Verification items for the finished model (mm, model axes). Face numbers are marked on the shaded views. Coordinates: 2 decimals unless noted, no trailing zeros. Order: outer loops, then holes, each group sorted by start corner. A loop starts at its lowest first (then second) coordinate and runs counter-clockwise, first axis right, second up. Notation, with made-up numbers: (-3.75, 73.25) - (47.25, 73.25) arc R6 ccw to (47.25, 82.25) - close; hole circle Ø2 at (74, 80.5). An arc over 180 degrees is marked (long way). One line per question, with ' | ' between items. Start each with the question number.
from build123d import *

# Parameters (mm, degrees)
SKETCH1_W           = 160
SKETCH1_H           = 22
BOSS_EXTRUDE1_DEPTH = 1.25
SKETCH2_W           = 160
SKETCH2_H           = 2.5
BOSS_EXTRUDE2_DEPTH = 4.5
SKETCH4_R           = 1.6
CUT_EXTRUDE1_DEPTH  = 3.5


with BuildPart() as part:
    # Sketch1 → Boss-Extrude1 (new body, symmetric)
    with BuildSketch(Plane(origin=(0, 0, 0), x_dir=(1, 0, 0), z_dir=(0, 1, 0))):
        with Locations((-1.081081081, -6.855855856)):
            Rectangle(SKETCH1_W, SKETCH1_H)
    extrude(amount=BOSS_EXTRUDE1_DEPTH, both=True)

    # Sketch2 → Boss-Extrude2 (add)
    with BuildSketch(Plane(origin=(0, 1.25, 0), x_dir=(1, 0, 0), z_dir=(0, 1, 0))):
        with Locations((-1.081081081, 2.894144144)):
            Rectangle(SKETCH2_W, SKETCH2_H)
        with Locations((-1.081081081, -16.605855856)):
            Rectangle(SKETCH2_W, SKETCH2_H)
    extrude(amount=BOSS_EXTRUDE2_DEPTH)

    # Sketch4 → Cut-Extrude1 (cut, through all)
    with BuildSketch(Plane(origin=(0, 1.25, 0), x_dir=(1, 0, 0), z_dir=(0, 1, 0))):
        with Locations((73.918918919, -3.355855856)):
            Circle(SKETCH4_R)
        with Locations((73.918918919, -10.355855856)):
            Circle(SKETCH4_R)
        with Locations((-76.081081081, -10.355855856)):
            Circle(SKETCH4_R)
        with Locations((-76.081081081, -3.355855856)):
            Circle(SKETCH4_R)
    extrude(amount=-CUT_EXTRUDE1_DEPTH, mode=Mode.SUBTRACT)


solid = part.part
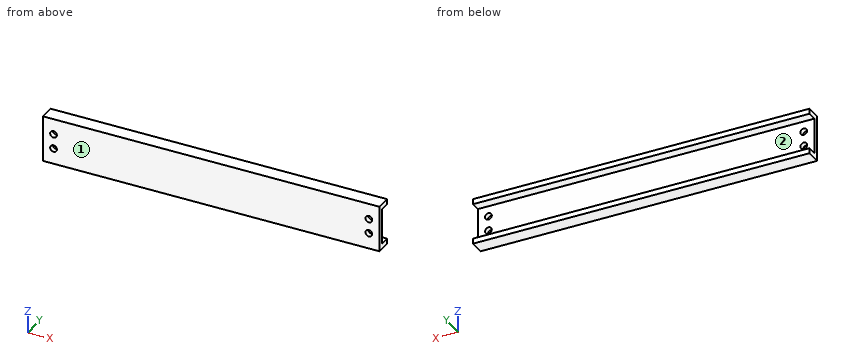
Item 1: Section check B-B (x = 60.5). Record the cut outline in (y, z), then the cut area to 3 significant figures.
Item 2: Section check C-C (z = 0). Record the cut outline in (x, y), then the cut area to 3 significant figures.
Item 3: Gauge pin test, flat end, axial feed: pin 1 (5 mm diameter, centred on x = 27, z = 3, fed in from +Y). Record the tip position at first contact, or that the pin passes through.
Item 4: Mould release check, pull along Z, two halves, no side actions. Record for the marked faces 1 and 2: +Z half, -Z half, draft (parallel to the pull), parting line (faces both ways), or undercut.
Item 5: Section check A-A (y = 4.25). Record the cut outline in (x, z), then the cut area to 3 significant figures.
Item 6: Thickness scan on probe 1 along X at (y, z) = (0.75, 3.25); probe 2 along Z at (x, y) = (-59, 1.5); probe 3 along X at (y, z) = (-0.5, 11.5). Record the ranges inside material, lowest first. Write a range as from..to.
Completed:
1) outline: (-1.25, -4.14) - (5.75, -4.14) - (5.75, -1.64) - (1.25, -1.64) - (1.25, 15.36) - (5.75, 15.36) - (5.75, 17.86) - (-1.25, 17.86) - close | area: 77.5 mm^2
2) outline: (-81.08, -1.25) - (78.92, -1.25) - (78.92, 1.25) - (-81.08, 1.25) - close | area: 400 mm^2
3) pin 1: stops at y = 1.25
4) face 1: draft | face 2: undercut
5) outline: (-81.08, -4.14) - (78.92, -4.14) - (78.92, -1.64) - (-81.08, -1.64) - close; (-81.08, 15.36) - (78.92, 15.36) - (78.92, 17.86) - (-81.08, 17.86) - close | area: 800 mm^2
6) probe 1: x = -81.08..-77.68, -74.48..72.32, 75.52..78.92 | probe 2: z = -4.14..-1.64, 15.36..17.86 | probe 3: x = -81.08..-77.2, -74.96..72.8, 75.04..78.92
